Can you work these out from the model? Positions are in its coordinate system, mm. Round coordinates to 2 decimals unless told otherwise and drop trailing zeros. Order: outer loops, then holes, each group sorted by start corner. A loop starts at its lowest first (then second) coordinate and runs counter-clockwise, first axis right, second up.
Q1. If I drill on line 1 (X direction, y = 4.25, z = -3.75); line 2 (Z direction, x = -21.5, y = -5.5); line 3 (Y direction, x = -16, z = 2.5), over which ranges is the centre line in solid material (lowest first)?
Q2. If we section it at C-C (x = -29): Please give me the cut outline in (y, z), plus the area to 3 significant figures.
Q3. Will these pins go through, and if not, where does the flat tip stop? P1, Ø1.5, axis at x = -7, z = -4.5, coming from the +Y side; P2, Ø1.5, axis at x = -13.5, z = 3, coming from the +Y side; P3, Ø3, axis at x = -16.5, y = -5.5, coming from the -Z side.
Q4. If we section it at B-B (x = -9): Please give me the cut outline in (y, z), plus the area to 3 significant figures.
from build123d import *


with BuildPart() as f1:
    # F0 (on Top) → F1 (revolve)
    with BuildSketch(Plane.XY):
        with BuildLine():
            Line((-31.75, 0), (0, 0))
            Line((0, 0), (0, 6.527945))
            ThreePointArc((0, 6.527945), (-0.309207, 7.072998), (-0.935696, 7.087236))
            ThreePointArc((-0.935696, 7.087236), (-11.833996, 4.448683), (-22.628869, 7.48276))
            ThreePointArc((-22.628869, 7.48276), (-22.866551, 7.564328), (-23.117263, 7.54731))
            ThreePointArc((-23.117263, 7.54731), (-27.034458, 6.987305), (-30.968462, 7.41349))
            ThreePointArc((-30.968462, 7.41349), (-31.50881, 7.293764), (-31.75, 6.795629))
            Line((-31.75, 6.795629), (-31.75, 0))
        make_face()
    revolve(axis=Axis((-15.875, 0, 0), (-1, 0, 0)))


solid = f1.part
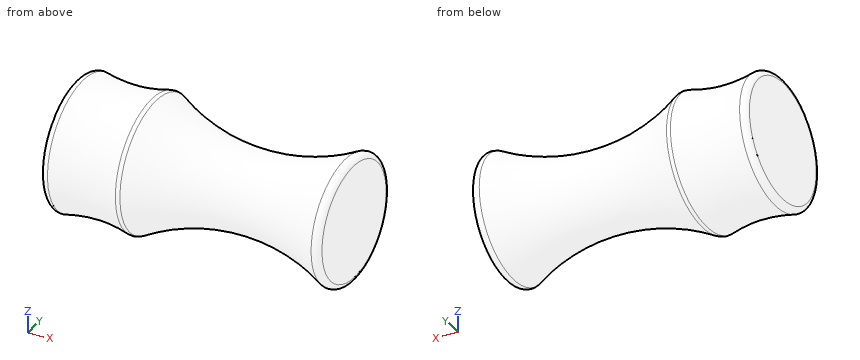
Solution:
1. line 1: x = -31.75 to -18.69, -4.17 to 0
1. line 2: z = -4.11 to 4.11
1. line 3: y = -4.24 to 4.24
2. outline: circle Ø14.15 at (0, 0)
2. area: 157 mm2
3. P1: stops at y = 3.17
3. P2: stops at y = 3.95
3. P3: stops at z = -3.15
4. outline: circle Ø9.16 at (0, 0)
4. area: 65.9 mm2
